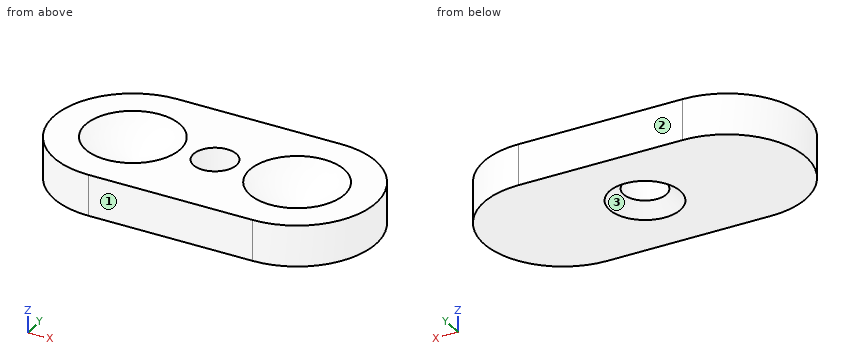
```python
from build123d import *

# Parameters (mm, degrees)
BOSS_EXTRUDE1_DEPTH                               = 3.302
CSK_FOR_4_FLAT_HEAD_MACHINE_SCREW_100_D           = 3.4544
CSK_FOR_4_FLAT_HEAD_MACHINE_SCREW_100_CSINK_D     = 5.715
CSK_FOR_4_FLAT_HEAD_MACHINE_SCREW_100_CSINK_ANGLE = 100


with BuildPart() as part:
    # Sketch1 → Boss-Extrude1 (new body)
    with BuildSketch(Plane.XY):
        with BuildLine():
            Line((-6.6675, 6.35), (6.6675, 6.35))
            ThreePointArc((6.6675, 6.35), (13.0175, 0), (6.6675, -6.35))
            Line((6.6675, -6.35), (-6.6675, -6.35))
            ThreePointArc((-6.6675, -6.35), (-13.0175, 0), (-6.6675, 6.35))
        make_face()
    extrude(amount=BOSS_EXTRUDE1_DEPTH)

    # Sketch4 → Cut-Revolve3 (revolve, cut)
    with BuildSketch(Plane(origin=(6.6675, 0, 0), x_dir=(0, 0, -1), z_dir=(1, 0, 0))):
        with BuildLine():
            Line((-3.302, 3.81), (-3.302, 0))
            Line((-3.302, 0), (-1.397, 0))
            ThreePointArc((-1.397, 0), (-2.038412152, 2.060543924), (-3.302, 3.81))
        make_face()
    cut_revolve3 = revolve(axis=Axis((6.6675, 0, 1.397), (0, 0, 1)), mode=Mode.SUBTRACT)

    # Mirror1: Cut-Revolve3 across plane
    add(cut_revolve3.mirror(Plane(origin=(0, 0, 0), x_dir=(0, 0, 1), z_dir=(1, 0, 0))), mode=Mode.SUBTRACT)

    # CSK for #4 Flat Head Machine Screw (100)1 (through all)
    with Locations(Plane(origin=(0, 0, 0), x_dir=(-1, 0, 0), z_dir=(0, 0, -1))):
        with Locations((0, 0)):
            CounterSinkHole(CSK_FOR_4_FLAT_HEAD_MACHINE_SCREW_100_D / 2, CSK_FOR_4_FLAT_HEAD_MACHINE_SCREW_100_CSINK_D / 2, counter_sink_angle=CSK_FOR_4_FLAT_HEAD_MACHINE_SCREW_100_CSINK_ANGLE)


solid = part.part
```
Here's how the part is built. I have some questions about the finished solid (model axes, mm). Face numbers are marked on the shaded views. Coordinates: 2 decimals unless noted, no trailing zeros. Loops run counter-clockwise (first coordinate to the right, second up) from the corner with the lowest first, then second, coordinate; pieces in that order, holes last. Notation, with made-up numbers: (63.25, 77) - (86.25, 77) arc R25 ccw to (86.25, 112) - close; hole circle Ø10 at (58, 37). An arc over 180 degrees is marked (long way). Return JSON: item names as keys, results as strings. Group by question number.
Item 1: If we section it at B-B on z = 2.1: State how many separate pieces and enclosed holes the cut face has, and give its area (3 significant figures).
Item 2: Will these pins go through, and if not, where does the flat tip stop? P1, Ø4.5, axis at x = 0, y = 0, coming from the -Z side; P2, Ø1.5, axis at x = -9.5, y = 1.5, coming from the -Z side.
Item 3: If we section it at A-A on x = 0: Write out the boundary of the cut face in (y, z), and give its area (3 significant figures).
Item 4: We'd pull the mould along Y, two halves only. Please class the marked faces 1, 2 and 3: +Y half, -Y half, draft (parallel to the pull), parting line (faces both ways), or undercut.
Item 5: I need wall thicknesses on line 1 (Y direction, x = 0, z = 1.4); line 2 (X direction, y = 0, z = 2). Which ranges of each line are inside material? Lowest first, please. Write a range as from..to.
Item 6: If we section it at C-C on x = -11: Write out the boundary of the cut face in (y, z), and give its area (3 significant figures).
Calculated:
{
 "1": {"separate pieces": "1", "enclosed holes": "3", "area": "257 mm^2"},
 "2": {"P1": "stops at z = 0.51", "P2": "stops at z = 0"},
 "3": {"outline": "(-6.35, 0) - (-2.86, 0) - (-1.73, 0.95) - (-1.73, 3.3) - (-6.35, 3.3) - close; (1.73, 0.95) - (2.86, 0) - (6.35, 0) - (6.35, 3.3) - (1.73, 3.3) - close", "area": "29.5 mm^2"},
 "4": {"face 1": "-Y half", "face 2": "+Y half", "face 3": "undercut"},
 "5": {"line 1": "y = -6.35..-1.73, 1.73..6.35", "line 2": "x = -13.02..-8.65, -4.69..-1.73, 1.73..4.69, 8.65..13.02"},
 "6": {"outline": "(-4.64, 0) - (4.64, 0) - (4.64, 3.3) - (-4.64, 3.3) - close", "area": "30.7 mm^2"}
}
